Input: part model. Units: mm. Frame: model coordinates. A direction names the side the tool comes from. Round coordinates to 2 decimals unless told otherwise and drop trailing zeros. Loops run counter-clockwise (first coordinate to the right, second up) from the corner with the lowest first, then second, coordinate; pieces in that order, holes last. Notation, with made-up numbers: (35, 64) - (85, 64) arc R16 cw to (85, 87) - close; hole circle Ø4 at (46, 30). An arc over 180 degrees is marked (long way). One line per question, with ' | ' between items. Start each with the question number.
Item 1: First-contact query: pin 1 (2 mm diameter, centred on x = 15, z = -1, fed in from -Y); pin 2 (3 mm diameter, centred on y = 8.5, z = -4, fed in from -X); pin 3 (1.5 mm diameter, centred on y = 59.5, z = -1.5, fed in from +X). Flat tips, straight axial feed; report the tip coordinate or a pass-through.
Item 2: Set-up query: faces 4 (the face through (30.057, 90.669, -5.395)), 5 (the face through (30, 90.7, -0.9)), 6 (the face through (-25, 98, 0)), 7 (the face through (-29, 87.4, -0.9)), 8 (the face through (-0.398, 201.928, -3.131)). Return all of +Z, -Z, +X, -X, +Y, -Y with unobstructed straight access to the full face (end or side cutting, diameter ignored); none if empty.
Item 3: Section A-A, the plane z = -5. Return loops of the section in (x, y), plus the area to 3 significant figures.
Item 4: Draft query along X for faces 1 (the face through (-29.056, 87.436, -5.395)), 2 (the face through (1.405, -24.368, -3.131)), 3 (the face through (-25, 98, -6.35)). Return one class per face: pulls with the +X half, pulls with the -X half, needs draft (parallel to the pull), parting line crosses it, or undercut.
Item 5: Material intervals for line 1 along Y through (x, z) = (11.5, -1.5); line 2 along X through (y, z) = (-16, -4.5); line 3 along X through (y, z) = (1, -1), sorted ascending.
Autodesk Inventor part; units mm, degrees
ref_plane "YZ Plane" through (0, 0, 0) normal (1, 0, 0) x (0, 1, 0)
ref_plane "XZ Plane" through (0, 0, 0) normal (0, 1, 0) x (-1, 0, 0)
ref_plane "XY Plane" through (0, 0, 0) normal (0, 0, 1) x (1, 0, 0)
sketch "Sketch1" plane through (0, 0, 0) normal (0, 0, 1) x (1, 0, 0)
  line L0 (25.7585, 0.0668) -> (23.5051, 178.1043)
  line L1 (-24.7511, 177.4935) -> (-22.4976, -0.544)
  line L2 (32.1011, 0.692) -> (29.8546, 178.1847)
  line L3 (-31.1006, 177.4131) -> (-28.854, -0.0795)
  arc A0 (29.8546, 178.1847) -> (-31.1006, 177.4131) centre (-0.623, 177.7989) ccw
  arc A1 (-28.854, -0.0795) -> (32.1011, 0.692) centre (1.6236, 0.3063) ccw
  arc A2 (-22.4976, -0.544) -> (25.7585, 0.0668) centre (1.6305, -0.2386) ccw
  arc A3 (23.5051, 178.1043) -> (-24.7511, 177.4935) centre (-0.623, 177.7989) ccw
  point P0 (0, 0)
  dimension "d6" = 6.35
  dimension "d7" = 6.35
  dimension "d11" = 177.8
  dimension "d12" = 177.8
  dimension "d13" = 24.13
extrude "Extrusion1" add sketch "Sketch1" against normal blind 6.35
fillet "Fillet1" radius 3.175 8 edges at (30.9778, 89.4384, 0) (-1.0088, 208.2765, 0) (-29.9773, 88.6668, 0) (2.0093, -30.1713, 0) (30.9778, 89.4384, -6.35) (-1.0088, 208.2765, -6.35) (-29.9773, 88.6668, -6.35) (2.0093, -30.1713, -6.35)
properties part number "7in polycord loop"
Return value:
1) pin 1: y = -27.02 | pin 2: x = -28.98 | pin 3: x = 31.22
2) face 4: -Z, +X, +Y | face 5: +Z, +X, +Y | face 6: +Z, +X, -X, +Y, -Y | face 7: +Z, -X, -Y | face 8: +Z, -Z
3) outline: (-30.52, 177.42) - (-28.28, -0.07) arc R29.9 ccw to (31.52, 0.68) - (29.28, 178.18) arc R29.9 ccw to start; hole (-24.75, 177.49) - (-22.5, -0.54) arc R24.13 ccw to (25.76, 0.07) - (23.51, 178.1) arc R24.13 ccw to start | area: 3,000 mm2
4) face 1: pulls with the -X half | face 2: undercut | face 3: needs draft
5) line 1: -28.02 to -22.26, 198.66 to 205.24 | line 2: -23.78 to -16.64, 19.9 to 27.03 | line 3: -28.01 to -22.52, 25.75 to 31.24
